Part model, mm, in its own coordinate system. Face numbers are marked on the shaded views. Give positions to 0.01 mm unless a question says otherwise; leave off trailing zeros. Write each loop counter-clockwise with the first axis right and the second up, starting at its lowest first coordinate (ties: lowest second). Pieces come first, ordered by that corner, then holes.
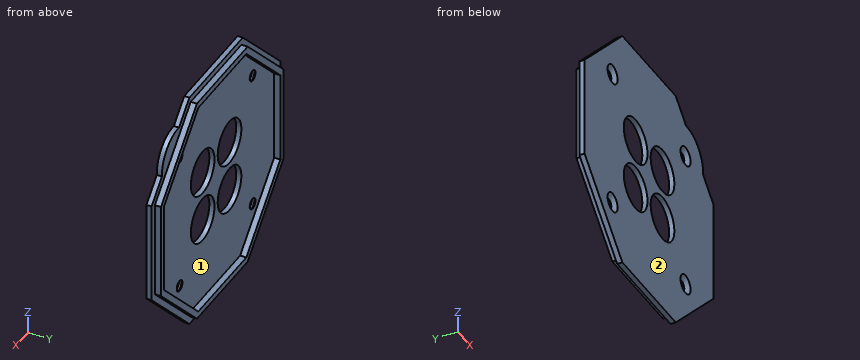
Autodesk Inventor part; units mm, degrees
ref_plane "YZ Plane" through (0, 0, 0) normal (1, 0, 0) x (0, 1, 0)
ref_plane "XZ Plane" through (0, 0, 0) normal (0, 1, 0) x (-1, 0, 0)
ref_plane "XY Plane" through (0, 0, 0) normal (0, 0, 1) x (1, 0, 0)
sketch "Skizze4" plane through (0, 0, 0) normal (0, 1, 0) x (-1, 0, 0)
  line L0 (24.8528, 60) -> (60, 24.8528)
  line L1 (60, 24.8528) -> (60, -24.8528)
  line L2 (60, -24.8528) -> (24.8528, -60)
  line L3 (24.8528, -60) -> (-24.8528, -60)
  line L4 (-24.8528, -60) -> (-60, -24.8528)
  line L5 (-60, -24.8528) -> (-60, 24.8528)
  line L6 (-60, 24.8528) -> (-24.8528, 60)
  line L7 (-24.8528, 60) -> (24.8528, 60)
  line L8 (0, -84) -> (0, 84) construction
  line L9 (84, 0) -> (-84, 0) construction
  point P0 (0, 0)
  point P1 (0, 0)
  dimension "d4" = 120
extrude "Extrusion2" add sketch "Skizze4" along normal blind 2.5
sketch "Skizze9" plane through (0, 2.5, 0) normal (0, 1, 0) x (1, 0, 0)
  line L0 (-60, -24.8528) -> (-24.8528, -60) construction
  line L1 (-24.8528, -60) -> (24.8528, -60) construction
  line L2 (24.8528, -60) -> (60, -24.8528) construction
  line L3 (60, -24.8528) -> (60, 24.8528) construction
  line L4 (60, 24.8528) -> (24.8528, 60) construction
  line L5 (24.8528, 60) -> (-24.8528, 60) construction
  line L6 (-24.8528, 60) -> (-60, 24.8528) construction
  line L7 (-60, 24.8528) -> (-60, -24.8528) construction
  line L8 (-23.6102, -57) -> (-57, -23.6102)
  line L9 (-57, -23.6102) -> (-57, 23.6102)
  line L10 (-57, 23.6102) -> (-23.6102, 57)
  line L11 (-23.6102, 57) -> (23.6102, 57)
  line L12 (23.6102, 57) -> (57, 23.6102)
  line L13 (57, 23.6102) -> (57, -23.6102)
  line L14 (57, -23.6102) -> (23.6102, -57)
  line L15 (23.6102, -57) -> (-23.6102, -57)
  line L16 (-54, -22.3675) -> (-22.3675, -54)
  line L17 (-22.3675, -54) -> (22.3675, -54)
  line L18 (22.3675, -54) -> (54, -22.3675)
  line L19 (54, -22.3675) -> (54, 22.3675)
  line L20 (54, 22.3675) -> (22.3675, 54)
  line L21 (22.3675, 54) -> (-22.3675, 54)
  line L22 (-22.3675, 54) -> (-54, 22.3675)
  line L23 (-54, 22.3675) -> (-54, -22.3675)
  point P0 (0, 0)
  dimension "d20" = 3
  dimension "d21" = 3
extrude "Extrusion6" add sketch "Skizze9" along normal blind 3
sketch "Skizze7" plane through (0, 0, 0) normal (0, -1, 0) x (1, 0, 0)
  line L0 (-24.8528, 60) -> (-60, 24.8528) construction
  line L1 (-60, 24.8528) -> (-60, -24.8528) construction
  line L2 (-60, -24.8528) -> (-24.8528, -60) construction
  line L3 (-24.8528, -60) -> (24.8528, -60) construction
  line L4 (24.8528, -60) -> (60, -24.8528) construction
  line L5 (60, -24.8528) -> (60, 24.8528) construction
  line L6 (60, 24.8528) -> (24.8528, 60)
  line L7 (24.8528, 60) -> (-24.8528, 60) construction
  line L8 (-84, 0) -> (84, 0) construction
  arc A0 (50.3321, 34.5207) -> (34.5207, 50.3321) centre (35.3553, 35.3553) ccw
  line L9 (35.3553, 35.3553) -> (49.4431, 49.4431) construction
  line L10 (50.3321, 34.5207) -> (34.5207, 50.3321) construction
  point P0 (0, 0)
  dimension "d61" = 10
  dimension "d62" = 15
  dimension "d63" = 49.7056
  dimension "d64" = 24.8528
extrude "Extrusion5" add sketch "Skizze7" against normal up to surface (2.5 mm away)
sketch "Skizze11" plane through (0, 0, 0) normal (0, -1, 0) x (1, 0, 0)
  line L0 (-84, 0) -> (84, 0) construction
  line L1 (0, -84) -> (0, 84) construction
  point P0 (0, 0)
  point P1 (-12.5, 12.5)
  point P2 (-12.5, -12.5)
  point P3 (12.5, -12.5)
  point P4 (12.5, 12.5)
  dimension "d27" = 12.5
  dimension "d31" = 12.5
  dimension "d34" = 360
hole "Bohrung1" at (-12.5, 0, 12.5) at (-12.5, 0, -12.5) at (12.5, 0, -12.5) at (12.5, 0, 12.5) direction (0, 1, 0) diameter 22 end through all
sketch "Skizze12" plane through (0, 0, 0) normal (0, -1, 0) x (1, 0, 0)
  line L0 (-24.8528, 60) -> (-60, 24.8528)
  line L1 (60, 24.8528) -> (24.8528, 60)
  line L2 (24.8528, -60) -> (60, -24.8528)
  line L3 (-60, -24.8528) -> (-24.8528, -60)
  line L4 (24.8528, 60) -> (24.8528, 24.8528) construction
  line L5 (24.8528, 24.8528) -> (60, 24.8528) construction
  line L6 (24.8528, 24.8528) -> (42.4264, 42.4264) construction
  line L7 (24.8528, 60) -> (-24.8528, 60) construction
  point P0 (0, 0)
  point P1 (33.9411, 33.9411)
  dimension "d44" = 12
  dimension "d47" = 45
hole "Bohrung2" at (33.9411, 0, 33.9411) direction (0, 1, 0) diameter 5.3 end through all
pattern_circular "Runde Anordnung1" count 4 over 360 about axis through (0, -10, 0) along (0, 1, 0) of "Bohrung2"
chamfer "Fase1" distance 2 angle 45 4 edges at (36.5911, 0, -33.9411) (33.9411, 0, 36.5911) (-36.5911, 0, 33.9411) (-33.9411, 0, -36.5911)
equation "\"d64\" = 0.5 * d63"
properties part number "Oktagon_Deckel" material "PC/ABS-Kunststoff"
1) Flat gauge pins, fed straight in: P1, Ø20, axis at x = 12.5, z = 12.5, coming from the -Y side; P2, Ø6, axis at x = -33.94, z = 33.94, coming from the +Y side; P3, Ø3, axis at y = 3, z = 41.5, coming from the -X side; P4, Ø7, axis at x = 33.94, z = 33.94, coming from the -Y side. Where does each tip first touch, or does it go through?
Check result:
P1: passes through
P2: stops at y = 2.5
P3: stops at x = -44.77
P4: stops at y = 1.15
2) Mould opens along X. For the marked faces 1 and 2 say: +X half, -X half, draft (parallel to the pull), parting line (faces both ways), or undercut.
Check result:
face 1: undercut
face 2: draft
3) Saw through at A-A (z = 12.5). Write the cut outline in (x, y), and give its area (3 significant figures).
Check result:
outline: (-60, 0) - (-23.5, 0) - (-23.5, 2.5) - (-54, 2.5) - (-54, 5.5) - (-57, 5.5) - (-57, 2.5) - (-60, 2.5) - close; (-1.5, 0) - (1.5, 0) - (1.5, 2.5) - (-1.5, 2.5) - close; (23.5, 0) - (60, 0) - (60, 2.5) - (57, 2.5) - (57, 5.5) - (54, 5.5) - (54, 2.5) - (23.5, 2.5) - close
area: 208 mm2
4) Saw through at D-D (x = -46.5). Write the cut outline in (y, z).
Check result:
outline: (0, -38.35) - (2.5, -38.35) - (2.5, -34.11) - (5.5, -34.11) - (5.5, -29.87) - (2.5, -29.87) - (2.5, 29.87) - (5.5, 29.87) - (5.5, 34.11) - (2.5, 34.11) - (2.5, 38.35) - (0, 38.35) - close
5) Saw through at C-C (z = 46.5). Write the cut outline in (x, y).
Check result:
outline: (-38.35, 0) - (45.4, 0) - (45.4, 2.5) - (34.11, 2.5) - (34.11, 5.5) - (29.87, 5.5) - (29.87, 2.5) - (-29.87, 2.5) - (-29.87, 5.5) - (-34.11, 5.5) - (-34.11, 2.5) - (-38.35, 2.5) - close
6) Drill centre lines: L1, parallel to Z at x = 12.5, y = 0.8; L2, parallel to X at y = 2.75, z = 7. Where is each one in solid material? Low to high.
Check result:
L1: z = -60 to -23.5, -1.5 to 1.5, 23.5 to 60
L2: x = -57 to -54, 54 to 57
7) Saw through at B-B (x = 12.5). Write the cut outline in (y, z), and give its area (3 significant figures).
Check result:
outline: (0, -60) - (2.5, -60) - (2.5, -57) - (5.5, -57) - (5.5, -54) - (2.5, -54) - (2.5, -23.5) - (0, -23.5) - close; (0, -1.5) - (2.5, -1.5) - (2.5, 1.5) - (0, 1.5) - close; (0, 23.5) - (2.5, 23.5) - (2.5, 54) - (5.5, 54) - (5.5, 57) - (2.5, 57) - (2.5, 60) - (0, 60) - close
area: 208 mm2
